```python
from build123d import *

# Parameters (mm, degrees)
SKETCH1_R           = 5
SKETCH1_R_2         = 2.75
BOSS_EXTRUDE1_DEPTH = 10
FILLET1_R           = 3


with BuildPart() as part:
    # Sketch1 → Boss-Extrude1 (new body)
    with BuildSketch(Plane.XY):
        Polygon((-21.5, -5), (-21.5, 5), (0, 10), (21.5, 5), (21.5, -5), (0, -10), align=None)
        Circle(SKETCH1_R, mode=Mode.SUBTRACT)
        with Locations((-16, 0)):
            Circle(SKETCH1_R_2, mode=Mode.SUBTRACT)
        with Locations((16, 0)):
            Circle(SKETCH1_R_2, mode=Mode.SUBTRACT)
    extrude(amount=BOSS_EXTRUDE1_DEPTH)

    # Fillet1
    fillet1_edges = [part.edges().sort_by_distance(p)[0] for p in [
        (21.5, 5, 5),
        (21.5, -5, 5),
        (0, -10, 5),
        (-21.5, -5, 5),
        (-21.5, 5, 5),
        (0, 10, 5),
    ]]
    fillet(fillet1_edges, radius=FILLET1_R)


solid = part.part
```
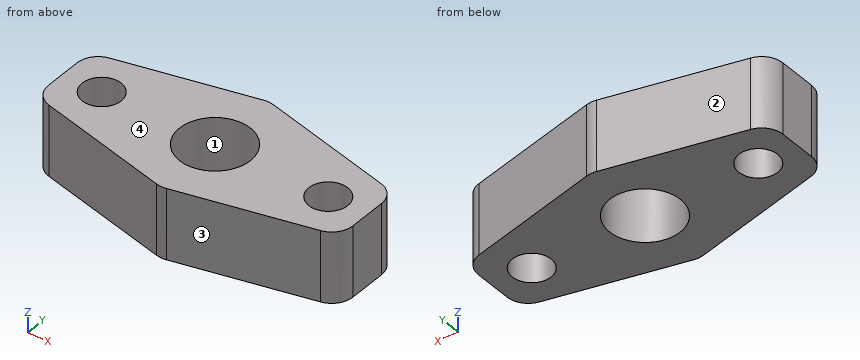
Could you check a few things on this model? Use its own coordinates, in mm. Face numbers are marked on the shaded views. Give positions to 0.01 mm unless a question says otherwise; leave off trailing zeros. Order: outer loops, then holes, each group sorted by start corner. A loop starts at its lowest first (then second) coordinate and runs counter-clockwise, first axis right, second up.
Q1. Suppose I cut it at A-A, the plane x = 0. Write out the boundary of the cut face in (y, z).
Q2. Suppose I cut it at D-D, the plane y = 4.25. Write out the boundary of the cut face in (x, z), and give its area (3 significant figures).
Q3. I'm going to push flat-ended pins straight in: P1, Ø1, axis at y = -5, z = 5, coming from the -X side; P2, Ø3, axis at x = 10.5, y = -2, coming from the -Z side; P3, Ø5, axis at x = 11, z = 1, coming from the -Y side; P4, Ø4, axis at x = 9.5, z = 3, coming from the -Y side. Where does each tip first touch, or does it pass through?
Q4. We'd pull the mould along X, two halves only. Please class the marked faces 1, 2, 3 and 4: +X half, -X half, draft (parallel to the pull), parting line (faces both ways), or undercut.
Q5. Suppose I cut it at B-B, the plane z = 1.5. Write out the boundary of the cut face in (x, y), and give its area (3 significant figures).
Q6. If I drill on line 1 along X through (y, z) = (1.5, 3.75); line 2 along X through (y, z) = (-2, 3); line 3 along Y through (x, z) = (-16, 7.5), over which ranges is the centre line in solid material (lowest first)?
Q7. Suppose I cut it at C-C, the plane y = 0. Write out the boundary of the cut face in (x, z), and give its area (3 significant figures).
Solution:
1. outline: (-9.92, 0) - (-5, 0) - (-5, 10) - (-9.92, 10) - close; (5, 0) - (9.92, 0) - (9.92, 10) - (5, 10) - close
2. outline: (-21.02, 0) - (-2.63, 0) - (-2.63, 10) - (-21.02, 10) - close; (2.63, 0) - (21.02, 0) - (21.02, 10) - (2.63, 10) - close
2. area: 368 mm2
3. P1: stops at x = -20.84
3. P2: stops at z = 0
3. P3: stops at y = -8.02
3. P4: stops at y = -8.26
4. face 1: undercut
4. face 2: -X half
4. face 3: +X half
4. face 4: draft
5. outline: (-21.5, -2.62) arc R3 ccw to (-19.18, -5.54) - (-0.68, -9.84) arc R3 ccw to (0.68, -9.84) - (19.18, -5.54) arc R3 ccw to (21.5, -2.62) - (21.5, 2.62) arc R3 ccw to (19.18, 5.54) - (0.68, 9.84) arc R3 ccw to (-0.68, 9.84) - (-19.18, 5.54) arc R3 ccw to (-21.5, 2.62) - close; hole circle Ø5.5 at (-16, 0); hole circle Ø10 at (0, 0); hole circle Ø5.5 at (16, 0)
5. area: 514 mm2
6. line 1: x = -21.5 to -18.3, -13.7 to -4.77, 4.77 to 13.7, 18.3 to 21.5
6. line 2: x = -21.5 to -17.89, -14.11 to -4.58, 4.58 to 14.11, 17.89 to 21.5
6. line 3: y = -6.28 to -2.75, 2.75 to 6.28
7. outline: (-21.5, 0) - (-18.75, 0) - (-18.75, 10) - (-21.5, 10) - close; (-13.25, 0) - (-5, 0) - (-5, 10) - (-13.25, 10) - close; (5, 0) - (13.25, 0) - (13.25, 10) - (5, 10) - close; (18.75, 0) - (21.5, 0) - (21.5, 10) - (18.75, 10) - close
7. area: 220 mm2
